Work out the finished part from the listing and answer in its coordinate system (mm). A direction names the side the tool comes from. Round coordinates to 2 decimals unless told otherwise and drop trailing zeros. Loops run counter-clockwise (first coordinate to the right, second up) from the corner with the lowest first, then second, coordinate; pieces in that order, holes last.
from build123d import *

# Parameters (mm, degrees)
F1_DEPTH = 373.5


with BuildPart() as f1:
    # F0 (on Top) → F1 (new body, symmetric)
    with BuildSketch(Plane.XY):
        with BuildLine():
            Line((2.5, -16.5), (9.5, -16.5))
            Line((9.5, -16.5), (9.5, -15))
            Line((9.5, -15), (2.5, -15))
            ThreePointArc((2.5, -15), (1.792893, -14.707107), (1.5, -14))
            Line((1.5, -14), (1.5, 14))
            ThreePointArc((1.5, 14), (1.792893, 14.707107), (2.5, 15))
            Line((2.5, 15), (14.5, 15))
            ThreePointArc((14.5, 15), (15.207107, 14.707107), (15.5, 14))
            Line((15.5, 14), (15.5, 5.5))
            Line((15.5, 5.5), (17, 5.5))
            Line((17, 5.5), (17, 14))
            ThreePointArc((17, 14), (16.267767, 15.767767), (14.5, 16.5))
            Line((14.5, 16.5), (2.5, 16.5))
            ThreePointArc((2.5, 16.5), (0.732233, 15.767767), (0, 14))
            Line((0, 14), (0, -14))
            ThreePointArc((0, -14), (0.732233, -15.767767), (2.5, -16.5))
        make_face()
    extrude(amount=F1_DEPTH, both=True)


solid = f1.part
Item 1: Each of these flat-tipped pins is pushed along its axis until it touches: P1, Ø0.8, axis at y = -15.5, z = 28.5, coming from the +X side; P2, Ø1.5, axis at x = 5.5, y = 13, coming from the +Z side; P3, Ø0.8, axis at x = 16, z = -143.5, coming from the -Y side. Where does it stop, or does it pass through?
Item 2: Section B-B, the plane y = -3 is taken. Give the vertices of the cut face in (x, z).
Item 3: Straight lines are drawn through the part: line 1 (Y direction, x = 6, z = 25); line 2 (X direction, y = 9.5, z = 204.5); line 3 (Y direction, x = 13.5, z = 124.5). For each, find the intervals that lie inside material, in ascending order.
Item 4: For faces 1 (the face through (1.5, 0, 5)), 2 (the face through (0, 0, 5)), determine the directions among +Z, -Z, +X, -X, +Y, -Y from which every point of the face is accessible in a straight line to the end or side of a thin tool.
Item 5: Determine the mould class of faces 3 (the face through (9, 16.5, 5)), 4 (the face through (8, 15, 5)), 5 (the face through (1, 3, -373.5)) for opening direction Y: pulls with the +Y half, pulls with the -Y half, needs draft (parallel to the pull), parting line crosses it, or undercut.
Item 6: Section A-A, the plane z = -310.5 is taken. Give the vertices of the cut face in (x, y), plus the area to 3 significant figures.
Answer below:
1. P1: stops at x = 9.5
1. P2: passes through
1. P3: stops at y = 5.5
2. outline: (0, -373.5) - (1.5, -373.5) - (1.5, 373.5) - (0, 373.5) - close
3. line 1: y = -16.5 to -15, 15 to 16.5
3. line 2: x = 0 to 1.5, 15.5 to 17
3. line 3: y = 15 to 16.5
4. face 1: +Z, -Z
4. face 2: +Z, -Z, -X, +Y, -Y
5. face 3: pulls with the +Y half
5. face 4: undercut
5. face 5: needs draft
6. outline: (0, -14) arc R2.5 ccw to (2.5, -16.5) - (9.5, -16.5) - (9.5, -15) - (2.5, -15) arc R1 cw to (1.5, -14) - (1.5, 14) arc R1 cw to (2.5, 15) - (14.5, 15) arc R1 cw to (15.5, 14) - (15.5, 5.5) - (17, 5.5) - (17, 14) arc R2.5 ccw to (14.5, 16.5) - (2.5, 16.5) arc R2.5 ccw to (0, 14) - close
6. area: 95.6 mm2
